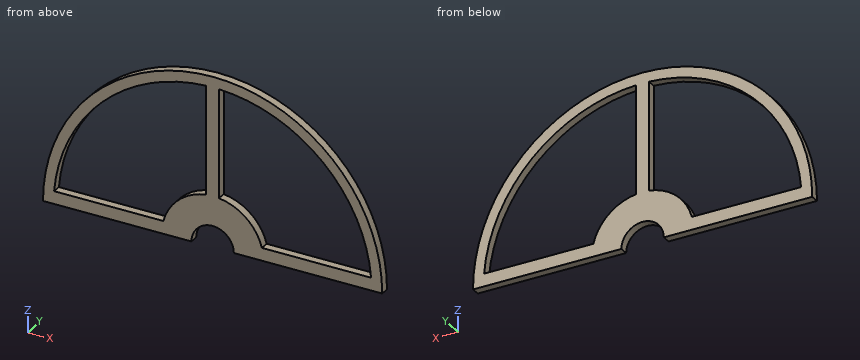
```python
from build123d import *

# Parameters (mm, degrees)
F0_R     = 80
F0_R_2   = 10
F1_DEPTH = 4
F2_R     = 75
F2_R_2   = 24
F3_DEPTH = 25
F4_W     = 3
F4_H     = 45
F5_DEPTH = 4
F6_W     = 170.305036
F6_H     = 83.79095
F7_DEPTH = 25


with BuildPart() as f1:
    # F0 (on Front) → F1 (new body)
    with BuildSketch(Plane.XZ):
        Circle(F0_R)
        Circle(F0_R_2, mode=Mode.SUBTRACT)
    extrude(amount=F1_DEPTH)

    # F2 (on face) → F3 (cut)
    with BuildSketch(Plane.XZ.offset(4)):
        Circle(F2_R)
        Circle(F2_R_2, mode=Mode.SUBTRACT)
    extrude(amount=-F3_DEPTH, mode=Mode.SUBTRACT)

    # F4 (on Front) → F5 (join)
    with BuildSketch(Plane.XZ):
        Polygon((17.140831, 6), (17.140831, 0), (76.595739, 0), (77.140831, 0), (77.140831, 6), align=None)
        with Locations((1.5, -43.351822)):
            Rectangle(F4_W, F4_H)
        with Locations((-1.5, -43.351822)):
            Rectangle(F4_W, F4_H)
        Polygon((-76.336667, 0), (-17.078082, 0), (-17.078082, 6), (-77.078082, 6), (-77.078082, 0), align=None)
        Polygon((3, 76.524103), (-3, 76.524103), (-3, 16.524103), (0, 16.524103), (3, 16.524103), align=None)
    extrude(amount=F5_DEPTH)

    # F6 (on Front) → F7 (cut)
    with BuildSketch(Plane.XZ):
        with Locations((2.269793, -41.895475)):
            Rectangle(F6_W, F6_H)
    extrude(amount=F7_DEPTH, mode=Mode.SUBTRACT)


solid = f1.part
```
Model file for the job. Use its own axes, mm. Coordinates: 2 decimals unless noted, no trailing zeros. Order: outer loops, then holes, each group sorted by start corner. A loop starts at its lowest first (then second) coordinate and runs counter-clockwise, first axis right, second up. Notation, with made-up numbers: M 31,49 L 70,49 A29 cw 70,71 Z; hole C 7.5,21.5 d11. An arc over 180 degrees is marked long. Answer as CSV lines item,"result".
(1) Flat gauge pins, fed straight in: pin 1 (1.2 mm diameter, centred on x = -38.5, y = -3, fed in from +Z); pin 2 (1.2 mm diameter, centred on y = -2.5, z = 60, fed in from -X). Where does each tip first touch, or does it go through?
Geometry says:
pin 1,"stops at z = 70.45"
pin 2,"stops at x = -53.59"
(2) Band-saw the part on B-B, the plane x = 53. List the corners of the cut face in (y, z).
Geometry says:
outline,"M -4,0 L 0,0 L 0,6 L -4,6 Z; M -4,53.07 L 0,53.07 L 0,59.92 L -4,59.92 Z"
(3) Wall check: line 1 along X through (y, z) = (-1.65, 35); line 2 along X through (y, z) = (-0.7, 63); line 3 along X through (y, z) = (-0.9, 6.5). Give the ranges that are in metal, low to high.
Geometry says:
line 1,"x = -71.94 to -66.33, -3 to 3, 66.33 to 71.94"
line 2,"x = -49.31 to -40.69, -3 to 3, 40.69 to 49.31"
line 3,"x = -79.74 to -74.72, -23.1 to -7.6, 7.6 to 23.1, 74.72 to 79.74"
(4) Band-saw the part on D-D, the plane x = 37. List the corners of the cut face in (y, z), then the cut area to 3 significant figures.
Geometry says:
outline,"M -4,0 L 0,0 L 0,6 L -4,6 Z; M -4,65.24 L 0,65.24 L 0,70.93 L -4,70.93 Z"
area,"46.8 mm2"
(5) Band-saw the part on C-C, the plane z = 68.5. List the corners of the cut face in (x, y).
Geometry says:
outline,"M -41.32,-4 L -30.54,-4 L -30.54,0 L -41.32,0 Z; M -3,-4 L 3,-4 L 3,0 L -3,0 Z; M 30.54,-4 L 41.32,-4 L 41.32,0 L 30.54,0 Z"
(6) Band-saw the part on A-A, the plane y = -3.2. List the corners of the cut face in (x, z).
Geometry says:
outline,"M -80,0 L -10,0 A10 cw 10,0 L 80,0 A80 ccw Z; hole M -74.76,6 L -23.24,6 A24 cw -3,23.81 L -3,74.94 A75 ccw Z; hole M 3,23.81 A24 cw 23.24,6 L 74.76,6 A75 ccw 3,74.94 Z"
